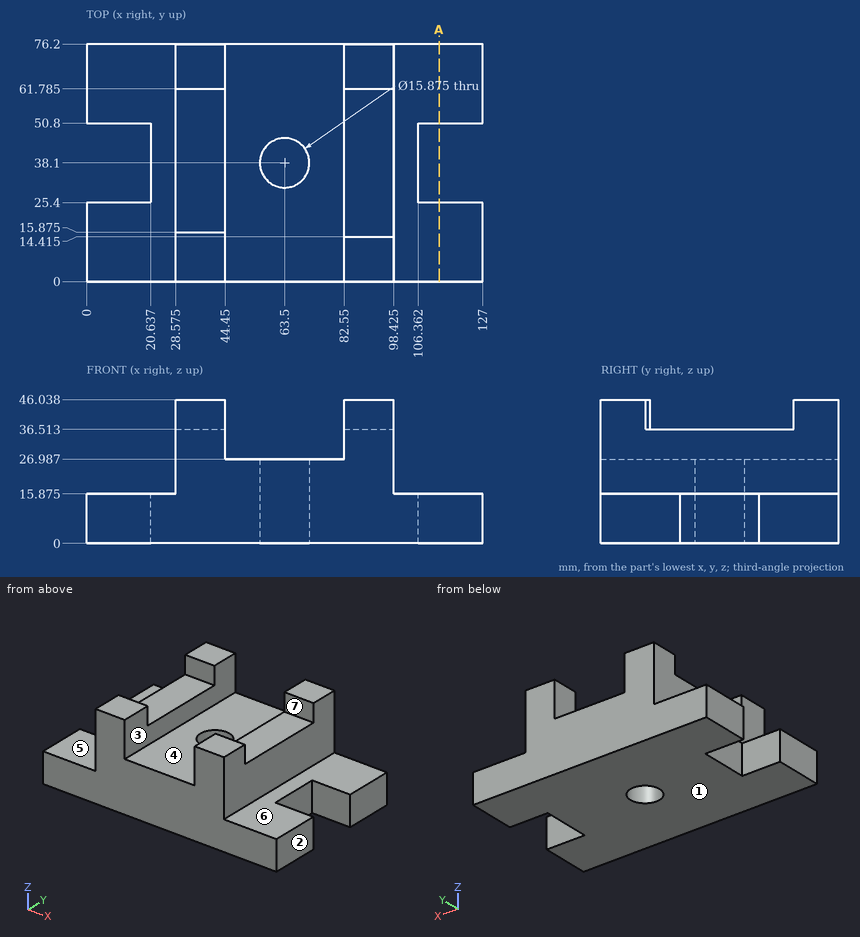
Could you check a few things on this drawing? It's one solid part, dimensions in mm from its lowest x, y, z. A direction names the side the tool comes from. Give positions to 0.01 mm unless a question says otherwise; leave off trailing zeros. Write each loop counter-clockwise with the first axis right and the second up, starting at its lowest first coordinate (ties: lowest second). Pieces come first, ordered by that corner, then holes. Notation, with made-up numbers: (19.25, 19.5) -> (74.25, 19.5) arc R23 cw to (74.25, 45.5) -> close; hole circle Ø5 at (-35.75, 60). An arc over 180 degrees is marked (long way). Answer as a JSON object with one key per item and string values.
Q1. Will these pins go through, and if not, where does the flat tip stop? pin 1 Ø5 at (x, y) = (89.5, 44.5) entering from +Z; pin 2 Ø2 at (x, y) = (62.5, 51) entering from +Z; pin 3 Ø14.5 at (x, y) = (13, 46.5) entering from +Z (1 decimal); pin 4 Ø8 at (x, z) = (91.5, 41) entering from -Y.
Taken from the geometry:
{"pin 1": "stops at z = 36.51", "pin 2": "stops at z = 26.99", "pin 3": "stops at z = 15.9", "pin 4": "stops at y = 0"}
Q2. We'd pull the mould along X, two halves only. Please class the marked faces 1, 2, 3 and 4: released by +X, released by -X, zero draft, split by the parting line, or undercut.
Taken from the geometry:
{"face 1": "zero draft", "face 2": "released by +X", "face 3": "undercut", "face 4": "undercut"}
Q3. Which directions (+Z, -Z, +X, -X, +Y, -Y) give clear straight access to the entire face, cutting with the end or side of a thin tool? Please do the marked faces 5, 6 and 7.
Taken from the geometry:
{"face 5": "+Z, -X, +Y, -Y", "face 6": "+Z, +X, +Y, -Y", "face 7": "+Z, +X, -X"}
Q4. Please list where these lines run through material, in increasing order: L1, parallel to Y at x = 63.5, z = 16.5; L2, parallel to X at y = 38, z = 8; L3, parallel to Y at x = 108, z = 11.5.
Taken from the geometry:
{"L1": "y = 0 to 30.16, 46.04 to 76.2", "L2": "x = 20.64 to 55.56, 71.44 to 106.36", "L3": "y = 0 to 25.4, 50.8 to 76.2"}
Q5. Suppose I cut it at A-A on x = 113. Write out the boundary of the cut face in (y, z) (1 decimal).
Taken from the geometry:
{"outline": "(0, 0) -> (25.4, 0) -> (25.4, 15.9) -> (0, 15.9) -> close; (50.8, 0) -> (76.2, 0) -> (76.2, 15.9) -> (50.8, 15.9) -> close"}
